CAD build for the part. Positions are in the model's coordinates, mm. A direction names the side the tool comes from. Round coordinates to 2 decimals unless told otherwise and drop trailing zeros. Loops run counter-clockwise (first coordinate to the right, second up) from the corner with the lowest first, then second, coordinate; pieces in that order, holes last. Notation, with made-up numbers: (-22.5, 61.5) -> (28.5, 61.5) arc R26 cw to (28.5, 94.5) -> close; hole circle Ø9 at (-8, 19). An arc over 180 degrees is marked (long way). Answer as CSV lines item,"result".
```python
from build123d import *

# Parameters (mm, degrees)
BOSS_EXTRUDE1_DEPTH = 3.175
BOSS_EXTRUDE2_DEPTH = 12.7
SKETCH3_W           = 6.604
SKETCH3_H           = 6.604
CUT_EXTRUDE1_DEPTH  = 77.145517599
SKETCH4_R           = 1.27
CUT_EXTRUDE3_DEPTH  = 25.4


with BuildPart() as part:
    # Sketch1 → Boss-Extrude1 (new body)
    with BuildSketch(Plane.XY):
        Polygon((-28.575, 19.594743879), (-19.594743879, 28.575), (19.594743879, 28.575), (28.575, 19.594743879), (28.575, -19.594743879), (19.594743879, -28.575), (-19.594743879, -28.575), (-28.575, -19.594743879), align=None)
    extrude(amount=BOSS_EXTRUDE1_DEPTH)

    # Sketch2 → Boss-Extrude2 (add)
    with BuildSketch(Plane.XY.offset(3.175)):
        with BuildLine():
            Line((-28.575, 19.594743879), (-19.594743879, 28.575))
            Line((-19.594743879, 28.575), (-4.490128061, 13.470384182))
            ThreePointArc((-4.490128061, 13.470384182), (0, 11.610512242), (4.490128061, 13.470384182))
            Line((4.490128061, 13.470384182), (19.594743879, 28.575))
            Line((19.594743879, 28.575), (28.575, 19.594743879))
            Line((28.575, 19.594743879), (13.470384182, 4.490128061))
            ThreePointArc((13.470384182, 4.490128061), (11.610512242, 0), (13.470384182, -4.490128061))
            Line((13.470384182, -4.490128061), (28.575, -19.594743879))
            Line((28.575, -19.594743879), (19.594743879, -28.575))
            Line((19.594743879, -28.575), (4.490128061, -13.470384182))
            ThreePointArc((4.490128061, -13.470384182), (0, -11.610512242), (-4.490128061, -13.470384182))
            Line((-4.490128061, -13.470384182), (-19.594743879, -28.575))
            Line((-19.594743879, -28.575), (-28.575, -19.594743879))
            Line((-28.575, -19.594743879), (-13.470384182, -4.490128061))
            ThreePointArc((-13.470384182, -4.490128061), (-11.610512242, 0), (-13.470384182, 4.490128061))
            Line((-13.470384182, 4.490128061), (-28.575, 19.594743879))
        make_face()
    extrude(amount=BOSS_EXTRUDE2_DEPTH)

    # Sketch3 → Cut-Extrude1 (cut, symmetric)
    with BuildSketch(Plane(origin=(24.084871939, 24.084871939, 0), x_dir=(0, 0, -1), z_dir=(0.7071067811865472, 0.7071067811865479, 0))):
        with Locations((-9.398, 0)):
            Rectangle(SKETCH3_W, SKETCH3_H)
    cut_extrude1 = extrude(amount=CUT_EXTRUDE1_DEPTH, both=True, mode=Mode.SUBTRACT)

    # Mirror1: Cut-Extrude1 across plane
    add(cut_extrude1.mirror(Plane.ZX), mode=Mode.SUBTRACT)

    # Sketch4 → Cut-Extrude3 (cut)
    with BuildSketch(Plane(origin=(0, 0, 0), x_dir=(-1, 0, 0), z_dir=(0, 0, -1))):
        with Locations((-19.594743879, 19.594743879)):
            Circle(SKETCH4_R)
        with Locations((-10.614487758, 10.614487758)):
            Circle(SKETCH4_R)
        with Locations((10.614487758, 10.614487758)):
            Circle(SKETCH4_R)
        with Locations((19.594743879, 19.594743879)):
            Circle(SKETCH4_R)
        with Locations((19.594743879, -19.594743879)):
            Circle(SKETCH4_R)
        with Locations((10.614487758, -10.614487758)):
            Circle(SKETCH4_R)
        with Locations((-19.594743879, -19.594743879)):
            Circle(SKETCH4_R)
        with Locations((-10.614487758, -10.614487758)):
            Circle(SKETCH4_R)
    extrude(amount=-CUT_EXTRUDE3_DEPTH, mode=Mode.SUBTRACT)


solid = part.part
```
Q1. Slice it at A-A, the plane z = 9.75. Give the cut face in (x, y) (3 decimals).
Results:
outline,"(-28.575, -19.595) -> (-26.42, -21.75) -> (-4.67, 0) -> (-26.42, 21.75) -> (-28.575, 19.595) -> (-13.47, 4.49) arc R6.35 cw to (-13.47, -4.49) -> close; (-21.75, -26.42) -> (-19.595, -28.575) -> (-4.49, -13.47) arc R6.35 cw to (4.49, -13.47) -> (19.595, -28.575) -> (21.75, -26.42) -> (0, -4.67) -> close; (-21.75, 26.42) -> (0, 4.67) -> (21.75, 26.42) -> (19.595, 28.575) -> (4.49, 13.47) arc R6.35 cw to (-4.49, 13.47) -> (-19.595, 28.575) -> close; (4.67, 0) -> (26.42, -21.75) -> (28.575, -19.595) -> (13.47, -4.49) arc R6.35 cw to (13.47, 4.49) -> (28.575, 19.595) -> (26.42, 21.75) -> close"
Q2. Drop flat-ended pins along their axis: pin 1 Ø3 at (x, y) = (-3, -19) entering from +Z (3 decimals); pin 2 Ø3 at (x, y) = (-22.5, 4.5) entering from -Z; pin 3 Ø6 at (x, z) = (-14.5, 7) entering from -Y; pin 4 Ø5 at (y, z) = (1, 8) entering from -X. Give the stop position or say it passes through.
Results:
pin 1,"z = 3.175"
pin 2,"z = 0"
pin 3,"y = -26.48"
pin 4,"x = -12.66"
Q3. Tool access for faces 4 (the flat face through (-11.94, -20.92, 9.44)), 5 (the flat face through (11.94, 20.92, 9.44)), 6 (the flat face through (-10.72, 15.39, 9.44)): list every direction of +Z, -Z, +X, -X, +Y, -Y with a clear straight run to the whole face (end or side of a thin tool).
Results:
face 4,"+Z, -Y"
face 5,"+Z, +Y"
face 6,"none"
Q4. Two-plate mould, pull along Z, no slides. Class faces 1 (the flat face through (0, 0, 0)), 2 (the flat face through (20.92, -11.94, 9.44)), 3 (the flat face through (15.7, 11.03, 9.44)): pulls with the +Z half, pulls with the -Z half, needs draft (parallel to the pull), parting line crosses it, or undercut.
Results:
face 1,"pulls with the -Z half"
face 2,"needs draft"
face 3,"undercut"
Q5. Probe L1, parallel to X at y = -7.5, z = 10.25; L2, parallel to Y at x = -9, z = 8.5; L3, parallel to X at y = 11, z = 3.75. List the from-to ranges inside material, lowest first. Write a range as [from, to].
Results:
L1,"[-16.48, -12.17], [-2.83, 2.83], [12.17, 16.48]"
L2,"[-17.98, -13.67], [-4.33, 4.33], [13.67, 17.98]"
L3,"[-19.98, -11.82], [-9.4, 9.4], [11.82, 19.98]"
Q6. Slice it at B-B, the plane y = 17.5. Give the cut face in (x, z) (3 decimals), and give its area (3 significant figures).
Results:
outline,"(-28.575, 0) -> (28.575, 0) -> (28.575, 3.175) -> (26.48, 3.175) -> (26.48, 15.875) -> (8.52, 15.875) -> (8.52, 3.175) -> (-8.52, 3.175) -> (-8.52, 15.875) -> (-26.48, 15.875) -> (-26.48, 3.175) -> (-28.575, 3.175) -> close; hole (-22.17, 6.096) -> (-12.83, 6.096) -> (-12.83, 12.7) -> (-22.17, 12.7) -> close; hole (12.83, 6.096) -> (22.17, 6.096) -> (22.17, 12.7) -> (12.83, 12.7) -> close"
area,"514 mm2"
Q7. Slice it at C-C, the plane y = -1. Give the cut face in (x, z) (3 decimals).
Results:
outline,"(-28.575, 0) -> (28.575, 0) -> (28.575, 3.175) -> (11.69, 3.175) -> (11.69, 15.875) -> (-11.69, 15.875) -> (-11.69, 3.175) -> (-28.575, 3.175) -> close; hole (-5.67, 6.096) -> (5.67, 6.096) -> (5.67, 12.7) -> (-5.67, 12.7) -> close"
Q8. Slice it at D-D, the plane x = 2. Give the cut face in (y, z) (3 decimals), and give its area (3 significant figures).
Results:
outline,"(-28.575, 0) -> (28.575, 0) -> (28.575, 3.175) -> (11.934, 3.175) -> (11.934, 15.875) -> (-11.934, 15.875) -> (-11.934, 3.175) -> (-28.575, 3.175) -> close; hole (-6.67, 6.096) -> (6.67, 6.096) -> (6.67, 12.7) -> (-6.67, 12.7) -> close"
area,"396 mm2"
